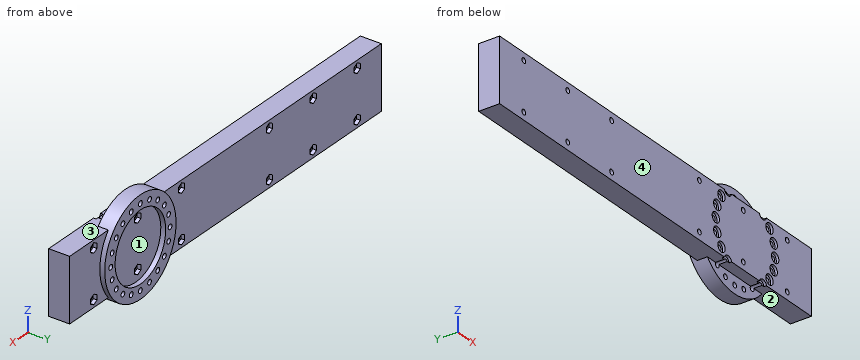
from build123d import *

# Parameters (mm, degrees)
SKETCH1_R                       = 32.5
BOSS_EXTRUDE1_DEPTH             = 10
SKETCH2_R                       = 23.05
CUT_EXTRUDE1_DEPTH              = 3.25
BOSS_EXTRUDE2_DEPTH             = 7.25
BOSS_EXTRUDE2_DEPTH_BACK        = 6.75
CBORE_FOR_M3_SBHCS1_D           = 3.4
CBORE_FOR_M3_SBHCS1_CBORE_D     = 6.7
CBORE_FOR_M3_SBHCS1_CBORE_DEPTH = 1.65
CUT_EXTRUDE3_DEPTH              = 2.5
SKETCH7_R                       = 1.7
CUT_EXTRUDE4_DEPTH              = 228.001789641


with BuildPart() as part:
    # Sketch1 → Boss-Extrude1 (new body)
    with BuildSketch(Plane(origin=(0, 0, 0), x_dir=(1, 0, 0), z_dir=(0, 1, 0))):
        with Locations(Location((0, 0, 0), (0, 0, 270))):
            Circle(SKETCH1_R)
    extrude(amount=BOSS_EXTRUDE1_DEPTH)

    # Sketch2 → Cut-Extrude1 (cut)
    with BuildSketch(Plane(origin=(0, 10, 0), x_dir=(1, 0, 0), z_dir=(0, 1, 0))):
        with Locations(Location((0, 0, 0), (0, 0, 270))):
            Circle(SKETCH2_R)
    extrude(amount=-CUT_EXTRUDE1_DEPTH, mode=Mode.SUBTRACT)

    # Sketch3 → Boss-Extrude2 (add, two sides: drawn at the far end of the back side and taken through both)
    with BuildSketch(Plane.XZ.offset(-BOSS_EXTRUDE2_DEPTH_BACK)):
        Polygon((-224, 21), (-3.439528279, 21), (60, 21), (60, -21), (-24.489517729, -21), (-224, -21), align=None)
    extrude(amount=BOSS_EXTRUDE2_DEPTH + BOSS_EXTRUDE2_DEPTH_BACK)

    # CBORE for M3 SBHCS1 (through all)
    with Locations(Plane.XZ.offset(7.25)):
        with Locations((0, 27.05), (8.358909698, 25.726078766), (15.899591075, 21.883909698), (21.883909698, 15.899591075), (25.726078766, 8.358909698), (27.05, 0), (25.726078766, -8.358909698), (21.883909698, -15.899591075), (15.899591075, -21.883909698), (8.358909698, -25.726078766), (0, -27.05), (-8.358909698, -25.726078766), (-15.899591075, -21.883909698), (-21.883909698, -15.899591075), (-25.726078766, -8.358909698), (-27.05, 0), (-25.726078766, 8.358909698), (-21.883909698, 15.899591075), (-15.899591075, 21.883909698), (-8.358909698, 25.726078766)):
            CounterBoreHole(CBORE_FOR_M3_SBHCS1_D / 2, CBORE_FOR_M3_SBHCS1_CBORE_D / 2, CBORE_FOR_M3_SBHCS1_CBORE_DEPTH)

    # Sketch6 → Cut-Extrude3 (cut)
    with BuildSketch(Plane(origin=(0, 6.75, 0), x_dir=(1, 0, 0), z_dir=(0, 1, 0))):
        Polygon((-202, 19.290896534), (-204.85, 17.645448267), (-204.85, 14.354551733), (-202, 12.709103466), (-199.15, 14.354551733), (-199.15, 17.645448267), align=None)
        Polygon((-202, -12.709103466), (-204.85, -14.354551733), (-204.85, -17.645448267), (-202, -19.290896534), (-199.15, -17.645448267), (-199.15, -14.354551733), align=None)
        Polygon((-162, -12.709103466), (-164.85, -14.354551733), (-164.85, -17.645448267), (-162, -19.290896534), (-159.15, -17.645448267), (-159.15, -14.354551733), align=None)
        Polygon((-122, -12.709103466), (-124.85, -14.354551733), (-124.85, -17.645448267), (-122, -19.290896534), (-119.15, -17.645448267), (-119.15, -14.354551733), align=None)
        Polygon((-162, 19.290896534), (-164.85, 17.645448267), (-164.85, 14.354551733), (-162, 12.709103466), (-159.15, 14.354551733), (-159.15, 17.645448267), align=None)
        Polygon((-122, 19.290896534), (-124.85, 17.645448267), (-124.85, 14.354551733), (-122, 12.709103466), (-119.15, 14.354551733), (-119.15, 17.645448267), align=None)
        Polygon((-42, 19.290896534), (-44.85, 17.645448267), (-44.85, 14.354551733), (-42, 12.709103466), (-39.15, 14.354551733), (-39.15, 17.645448267), align=None)
        Polygon((-2, 19.290896534), (-4.85, 17.645448267), (-4.85, 14.354551733), (-2, 12.709103466), (0.85, 14.354551733), (0.85, 17.645448267), align=None)
        Polygon((38, 19.290896534), (35.15, 17.645448267), (35.15, 14.354551733), (38, 12.709103466), (40.85, 14.354551733), (40.85, 17.645448267), align=None)
        Polygon((38, -12.709103466), (35.15, -14.354551733), (35.15, -17.645448267), (38, -19.290896534), (40.85, -17.645448267), (40.85, -14.354551733), align=None)
        Polygon((-2, -12.709103466), (-4.85, -14.354551733), (-4.85, -17.645448267), (-2, -19.290896534), (0.85, -17.645448267), (0.85, -14.354551733), align=None)
        Polygon((-42, -12.709103466), (-44.85, -14.354551733), (-44.85, -17.645448267), (-42, -19.290896534), (-39.15, -17.645448267), (-39.15, -14.354551733), align=None)
    extrude(amount=-CUT_EXTRUDE3_DEPTH, mode=Mode.SUBTRACT)

    # Sketch7 → Cut-Extrude4 (cut, through all)
    with BuildSketch(Plane.XZ.offset(7.25)):
        with Locations(Location((-202, 16, 0), (0, 0, 270))):
            Circle(SKETCH7_R)
        with Locations(Location((-202, -16, 0), (0, 0, 270))):
            Circle(SKETCH7_R)
        with Locations(Location((-162, -16, 0), (0, 0, 270))):
            Circle(SKETCH7_R)
        with Locations(Location((-162, 16, 0), (0, 0, 270))):
            Circle(SKETCH7_R)
        with Locations(Location((-122, 16, 0), (0, 0, 270))):
            Circle(SKETCH7_R)
        with Locations(Location((-122, -16, 0), (0, 0, 270))):
            Circle(SKETCH7_R)
        with Locations(Location((-42, 16, 0), (0, 0, 270))):
            Circle(SKETCH7_R)
        with Locations(Location((-2, 16, 0), (0, 0, 270))):
            Circle(SKETCH7_R)
        with Locations(Location((38, 16, 0), (0, 0, 270))):
            Circle(SKETCH7_R)
        with Locations(Location((38, -16, 0), (0, 0, 270))):
            Circle(SKETCH7_R)
        with Locations(Location((-2, -16, 0), (0, 0, 270))):
            Circle(SKETCH7_R)
        with Locations(Location((-42, -16, 0), (0, 0, 270))):
            Circle(SKETCH7_R)
    extrude(amount=-CUT_EXTRUDE4_DEPTH, mode=Mode.SUBTRACT)


solid = part.part
Build history of the part. All positions in model axes, mm. Face numbers are marked on the shaded views. A direction names the side the tool comes from. Coordinates: 2 decimals unless noted, no trailing zeros. Order: outer loops, then holes, each group sorted by start corner. A loop starts at its lowest first (then second) coordinate and runs counter-clockwise, first axis right, second up. Notation, with made-up numbers: M 27.25,86 L 81.25,86 A12 cw 81.25,107 Z; hole C 88,32 d3. An arc over 180 degrees is marked long. One line per question, with ' | ' between items. Start each with the question number.
Q1. Saw through at A-A (x = -188). List the corners of the cut face in (y, z).
Q2. Probe L1, parallel to Z at x = -202, y = 1.5; L2, parallel to Z at x = 27.05, y = -6.7; L3, parallel to X at y = 9.25, z = -16.5. List the from-to ranges inside material, lowest first. Write a range as from..to.
Q3. Flat gauge pins, fed straight in: pin 1 Ø2 at (x, z) = (23.5, 16.5) entering from -Y; pin 2 Ø5 at (x, z) = (-192.5, -11.5) entering from +Y; pin 3 Ø10 at (x, y) = (8, -4) entering from +Z. Where does each tip first touch, or does it go through?
Q4. 3-axis set-ups, long thin cutter, end or side, ignore diameter. For the marked faces 1, 2, 3 and 4: which of +Z, -Z, +X, -X, +Y, -Y reach the whole face in a straight line?
Check values:
1) outline: M -7.25,-21 L 6.75,-21 L 6.75,21 L -7.25,21 Z
2) L1: z = -21..-17.7, -14.3..14.3, 17.7..21 | L2: z = -21..-11.44, -5.28..-3.35, 3.35..5.28, 11.44..21 | L3: x = -28..-23.47, -20.29..-16.1, 16.1..20.29, 23.47..28
3) pin 1: stops at y = -5.6 | pin 2: stops at y = 6.75 | pin 3: stops at z = 32.11
4) face 1: +Y | face 2: -Z, +X, -Y | face 3: +Z, +X, -Y | face 4: +Z, -Z, +X, -X, -Y
